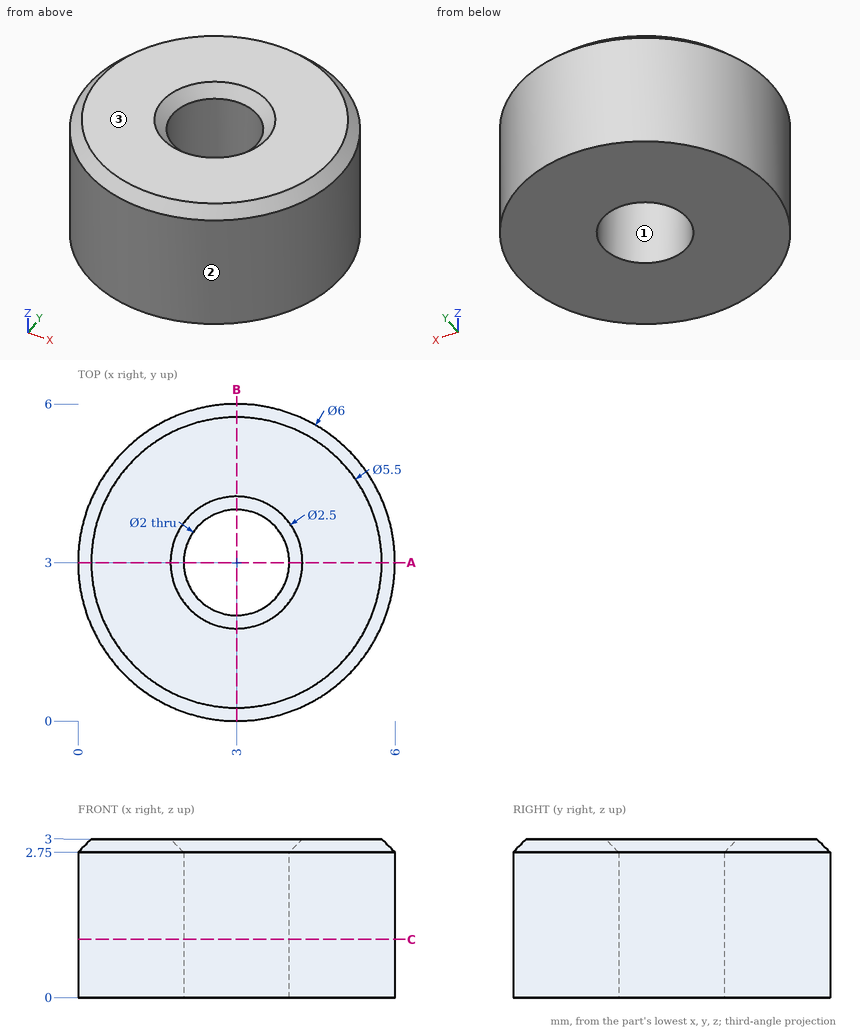
Here's the drawing with two shaded views (mm, measured from the low corner). I have some questions. Coordinates: 2 decimals unless noted, no trailing zeros. Loops run counter-clockwise (first coordinate to the right, second up) from the corner with the lowest first, then second, coordinate; pieces in that order, holes last. Notation, with made-up numbers: M 74,65 L 120,65 A24 ccw 120,90 Z; hole C -22,65 d5. An arc over 180 degrees is marked long. Answer as CSV lines item,"result". Start each with the question number.
1. Suppose I cut it at C-C, the plane z = 1.1. List the corners of the cut face in (x, y) for me.
2. Thinking about a two-plate mould opening in X: for the marked faces 1, 2 and 3, which applies, +X half, -X half, draft (parallel to the pull), parting line (faces both ways), or undercut?
3. Suppose I cut it at A-A, the plane y = 3. List the corners of the cut face in (x, z) for me.
4. If I drill on probe 1 along Y at (x, z) = (3, 1.5); probe 2 along Z at (x, y) = (1.15, 5.2); probe 3 along X at (y, z) = (0.45, 1.05), over which ranges is the centre line in solid material (lowest first)? Write a range as [from, to].
5. For pin 1 Ø1 at (x, z) = (5, 1) entering from +Y, with a flat end and sliding along its axis, tell me the tip position at first contact or that it passes through.
Output:
1,outline,"C 3,3 d6; hole C 3,3 d2"
2,face 1,"undercut"
2,face 2,"parting line"
2,face 3,"draft"
3,outline,"M 0,0 L 2,0 L 2,2.75 L 1.75,3 L 0.25,3 L 0,2.75 Z; M 4,0 L 6,0 L 6,2.75 L 5.75,3 L 4.25,3 L 4,2.75 Z"
4,probe 1,"y = [0, 2], [4, 6]"
4,probe 2,"z = [0, 2.88]"
4,probe 3,"x = [1.42, 4.58]"
5,pin 1,"stops at y = 5.6"
